Geometry check sheet. Reference: the model listing, model coordinates, mm. Give positions to 0.01 mm unless a question says otherwise; leave off trailing zeros. Order: outer loops, then holes, each group sorted by start corner. A loop starts at its lowest first (then second) coordinate and runs counter-clockwise, first axis right, second up. Notation, with made-up numbers: M 8.25,-35 L 60.25,-35 A32 cw 60.25,-8 Z; hole C 23,-36.5 d7. An arc over 180 degrees is marked long. Put each result on its own line as item: value. Start each with the question number.
Q1. Material ranges on L1, parallel to X at y = 4.75, z = 1.45; L2, parallel to Y at x = 4, z = 1.05; L3, parallel to X at y = 0, z = 0.85, recorded low to high.
Q2. Section check A-A on z = 0.8. Record the cut outline in (x, y) (3 decimals), then the cut area to 3 significant figures.
Q3. Mould release check, pull along X, two halves, no side actions. Record for faces 1 (the cylindrical face through (-4.188, -4.206, 0.74)), 2 (the flat face through (6, 4, 1.5)), 3 (the flat face through (9.221, 10.803, 0.74)), 4 (the cylindrical face through (-4.144, 11.181, 0.74)): +X half, -X half, draft (parallel to the pull), parting line (faces both ways), or undercut.
Q4. Section check B-B on x = 13.5. Record the cut outline in (y, z), then the cut area to 3 significant figures.
Q5. Section check C-C on y = -2. Record the cut outline in (x, z).
Q6. Go/stop test with a flat-tipped pin: pin 1 (5 mm diameter, centred on x = 11, y = 5.5, fed in from -Z). Record where the tip stops, or that it passes through.
```python
from build123d import *

# Parameters (mm, degrees)
SKETCH1_R           = 0.5
BOSS_EXTRUDE1_DEPTH = 1.5


with BuildPart() as part:
    # Sketch1 → Boss-Extrude1 (new body)
    with BuildSketch(Plane.XY):
        with BuildLine():
            Line((12.364948684, 9.687701301), (5.987177096, 11.949653903))
            ThreePointArc((5.987177096, 11.949653903), (1.571990001, 12.356697641), (-2.501744354, 10.606197685))
            ThreePointArc((-2.501744354, 10.606197685), (-4.166324297, 11.161284148), (-3.73571139, 9.4602492))
            ThreePointArc((-3.73571139, 9.4602492), (-6.02117945, 3.467331645), (-3.73571139, -2.525585911))
            ThreePointArc((-3.73571139, -2.525585911), (-4.166324297, -4.226620858), (-2.501744354, -3.671534395))
            ThreePointArc((-2.501744354, -3.671534395), (1.571990001, -5.422034351), (5.987177096, -5.014990613))
            Line((5.987177096, -5.014990613), (12.364948684, -2.753038011))
            ThreePointArc((12.364948684, -2.753038011), (15.297909656, -0.673895607), (16.706003649, 2.634028895))
            ThreePointArc((16.706003649, 2.634028895), (18.25882055, 3.467331645), (16.706003649, 4.300634395))
            ThreePointArc((16.706003649, 4.300634395), (15.297909656, 7.608558897), (12.364948684, 9.687701301))
        make_face()
        with Locations((-3.485834311, 10.428526767)):
            Circle(SKETCH1_R, mode=Mode.SUBTRACT)
        with Locations((-3.485834311, -3.493863477)):
            Circle(SKETCH1_R, mode=Mode.SUBTRACT)
        with Locations((17.25882055, 3.467331645)):
            Circle(SKETCH1_R, mode=Mode.SUBTRACT)
    extrude(amount=BOSS_EXTRUDE1_DEPTH)


solid = part.part
```
Results found:
1. L1: x = -5.93 to 16.63
1. L2: y = -5.47 to 12.41
1. L3: x = -5.33 to 15.77
2. outline: M -3.736,-2.526 A1 ccw long -2.502,-3.672 A9 ccw 5.987,-5.015 L 12.365,-2.753 A6.6 ccw 16.706,2.634 A1 ccw long 16.706,4.301 A6.6 ccw 12.365,9.688 L 5.987,11.95 A9 ccw -2.502,10.606 A1 ccw long -3.736,9.46 A9 ccw Z; hole C -3.486,-3.494 d1; hole C -3.486,10.429 d1; hole C 17.259,3.467 d1
2. area: 319 mm^2
3. face 1: undercut
3. face 2: draft
3. face 3: +X half
3. face 4: undercut
4. outline: M -2.22,0 L 9.16,0 L 9.16,1.5 L -2.22,1.5 Z
4. area: 17.1 mm^2
5. outline: M -4.17,0 L 13.86,0 L 13.86,1.5 L -4.17,1.5 Z
6. pin 1: stops at z = 0
